```python
from build123d import *

# Parameters (mm, degrees)
F0_R     = 3.175
F1_DEPTH = 3.048


with BuildPart() as f1:
    # F0 (on Front) → F1 (new body)
    with BuildSketch(Plane.XZ):
        with BuildLine():
            ThreePointArc((9.394944, 112.731355), (9.49243, 113.512986), (9.525, 114.3))
            ThreePointArc((9.525, 114.3), (-0.787014, 123.79243), (-9.394944, 112.731355))
            ThreePointArc((-9.394944, 112.731355), (0, 104.775), (9.394944, 112.731355))
        make_face()
        with Locations((0, 114.3)):
            Circle(F0_R, mode=Mode.SUBTRACT)
        with BuildLine():
            ThreePointArc((9.394944, 112.731355), (0, 104.775), (-9.394944, 112.731355))
            Line((-9.394944, 112.731355), (-15.733267, 65.616587))
            ThreePointArc((-15.733267, 65.616587), (0, 79.375), (15.733267, 65.616587))
            Line((15.733267, 65.616587), (9.394944, 112.731355))
        make_face()
        with Locations((-1.5875, 93.633412)):
            Circle(F0_R, mode=Mode.SUBTRACT)
        with BuildLine():
            ThreePointArc((15.733267, 65.616587), (0, 79.375), (-15.733267, 65.616587))
            ThreePointArc((-15.733267, 65.616587), (-15.854012, 62.683953), (-15.432802, 59.779214))
            ThreePointArc((-15.432802, 59.779214), (0, 47.625), (15.432802, 59.779214))
            ThreePointArc((15.432802, 59.779214), (15.764063, 61.626515), (15.875, 63.5))
            ThreePointArc((15.875, 63.5), (15.839527, 64.560664), (15.733267, 65.616587))
        make_face()
        with Locations((0, 63.5)):
            Circle(F0_R, mode=Mode.SUBTRACT)
        with BuildLine():
            ThreePointArc((15.432802, 59.779214), (0, 47.625), (-15.432802, 59.779214))
            Line((-15.432802, 59.779214), (-6.94853, 6.514872))
            ThreePointArc((-6.94853, 6.514872), (3.502919, 8.857493), (9.525, 0))
            ThreePointArc((9.525, 0), (7.748219, -5.539921), (3.080754, -9.013023))
            Line((3.080754, -9.013023), (44.655779, -7.934832))
            ThreePointArc((44.655779, -7.934832), (36.5125, 0), (44.655779, 7.934832))
            Line((44.655779, 7.934832), (16.401671, 8.667563))
            ThreePointArc((16.401671, 8.667563), (10.493739, 11.533341), (8.756557, 17.865682))
            Line((8.756557, 17.865682), (15.432802, 59.779214))
        make_face()
        with BuildLine():
            ThreePointArc((9.525, 0), (3.502919, 8.857493), (-6.94853, 6.514872))
            ThreePointArc((-6.94853, 6.514872), (-8.001175, -5.167864), (3.080754, -9.013023))
            ThreePointArc((3.080754, -9.013023), (7.748219, -5.539921), (9.525, 0))
        make_face()
        Circle(F0_R, mode=Mode.SUBTRACT)
        with BuildLine():
            ThreePointArc((44.655779, 7.934832), (36.5125, 0), (44.655779, -7.934832))
            ThreePointArc((44.655779, -7.934832), (50.134948, -5.539429), (52.3875, 0))
            ThreePointArc((52.3875, 0), (50.134948, 5.539429), (44.655779, 7.934832))
        make_face()
        with Locations((44.45, 0)):
            Circle(F0_R, mode=Mode.SUBTRACT)
    extrude(amount=F1_DEPTH)


solid = f1.part
```
Source: CAD feature listing. Evaluate the final solid. Frame: model axes, mm. A direction names the side the tool comes from. Give positions to 0.01 mm unless a question says otherwise; leave off trailing zeros. Write each loop counter-clockwise with the first axis right and the second up, starting at its lowest first coordinate (ties: lowest second). Pieces come first, ordered by that corner, then holes.
1. First-contact query: pin 1 (1.5 mm diameter, centred on y = -1, z = 80, fed in from -X); pin 2 (1.5 mm diameter, centred on x = 17.5, y = -1, fed in from -Z). Flat tips, straight axial feed; report the tip coordinate or a pass-through.
2. Section query A-A (x = 0). Return the cut outline in (y, z) (3 decimals), then the cut area to 3 significant figures.
3. Pull-direction query (Z, two-part tool) for faces 4 (the face through (-15.856, -1.503, 62.725)), 5 (the face through (15.76, -1.5, 61.6)), 6 (the face through (3, 0, 58)); classes: +Z half, -Z half, draft (parallel to the pull), parting line (faces both ways), or undercut.
4. Material intervals for line 1 along Z through (x, y) = (44.45, -1.05) (3 decimals); line 2 along Z through (x, y) = (2.5, -2.8); line 3 along Z through (x, y) = (-2, -0.55), sorted ascending.
5. Section query B-B (x = 43). Return the cut outline in (y, z).
6. Access query for faces 1 (the face through (-11.25, -1.5, 33.52)), 2 (the face through (-0.69, -1.5, 111.2)), 3 (the face through (12.05, -1.5, 38.53)). Directions: +Z, -Z, +X, -X, +Y, -Y. A direction counts if a zero-diameter tool reaches every point of the face in a straight line with its end or side. Return the directions, or none.
7. Section query D-D (z = 52.5). Return the cut outline in (x, y).
8. Section query C-C (y = -0.8). Count the separate pieces of the cut face and the enclosed holes in it, then the cut area to 3 significant figures.
Output values:
1. pin 1: stops at x = -13.9
1. pin 2: stops at z = -8.66
2. outline: (-3.048, -9.525) - (0, -9.525) - (0, -3.175) - (-3.048, -3.175) - close; (-3.048, 3.175) - (0, 3.175) - (0, 60.325) - (-3.048, 60.325) - close; (-3.048, 66.675) - (0, 66.675) - (0, 90.884) - (-3.048, 90.884) - close; (-3.048, 96.383) - (0, 96.383) - (0, 111.125) - (-3.048, 111.125) - close; (-3.048, 117.475) - (0, 117.475) - (0, 123.825) - (-3.048, 123.825) - close
2. area: 332 mm2
3. face 4: parting line
3. face 5: undercut
3. face 6: draft
4. line 1: z = -7.94 to -3.175, 3.175 to 7.94
4. line 2: z = -9.19 to -1.96, 1.96 to 61.54, 65.46 to 112.34, 116.26 to 123.49
4. line 3: z = -9.31 to -2.47, 2.47 to 61.03, 65.97 to 90.49, 96.78 to 111.83, 116.77 to 123.61
5. outline: (-3.05, -7.98) - (0, -7.98) - (0, -2.82) - (-3.05, -2.82) - close; (-3.05, 2.82) - (0, 2.82) - (0, 7.98) - (-3.05, 7.98) - close
6. face 1: -X, +Y, -Y
6. face 2: +Y, -Y
6. face 3: +X, +Y, -Y
7. outline: (-14.27, -3.05) - (14.27, -3.05) - (14.27, 0) - (-14.27, 0) - close
8. separate pieces: 1
8. enclosed holes: 5
8. area: 3,560 mm2
